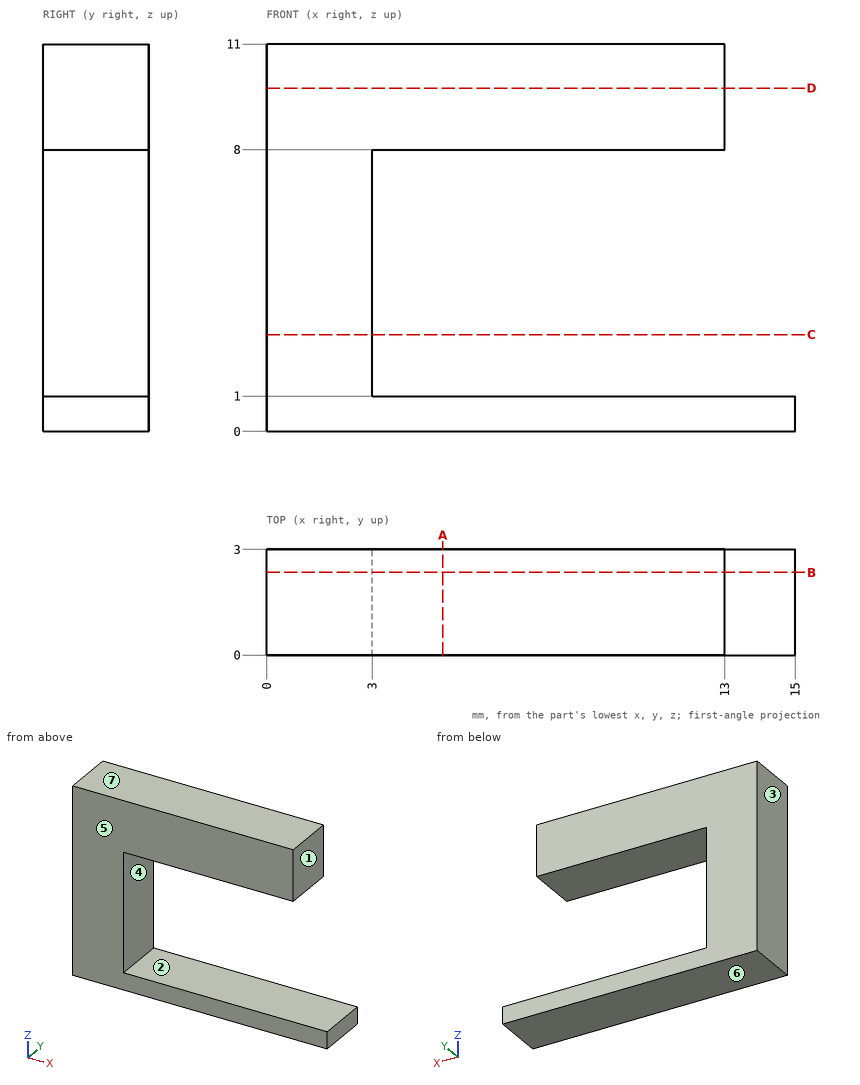
Geometry check sheet. Reference: drawing and pictorial views, mm from the part's lowest x, y, z. A direction names the side the tool comes from. Round coordinates to 2 decimals unless told otherwise and drop trailing zeros. Loops run counter-clockwise (first coordinate to the right, second up) from the corner with the lowest first, then second, coordinate; pieces in that order, holes last. Notation, with made-up numbers: (-27.5, 38.5) - (-3.5, 38.5) arc R25 ccw to (-3.5, 61.5) - close; hole circle Ø3 at (64.5, 88). An arc over 180 degrees is marked (long way). Use a Markdown table: item, result.
Q1. Cross-section at B-B on y = 2.35. Record the cut outline in (x, z).
Solutions:
| item | result |
|---|---|
| outline | (0, 0) - (15, 0) - (15, 1) - (3, 1) - (3, 8) - (13, 8) - (13, 11) - (0, 11) - close |
Q2. Go/stop test with a flat-tipped pin: P1, Ø0.9, axis at y = 2, z = 9.5, coming from the +X side. Record where the tip stops, or that it passes through.
Solutions:
| item | result |
|---|---|
| P1 | stops at x = 13 |
Q3. Cross-section at D-D on z = 9.75. Record the cut outline in (x, y).
Solutions:
| item | result |
|---|---|
| outline | (0, 0) - (13, 0) - (13, 3) - (0, 3) - close |
Q4. Cross-section at C-C on z = 2.75. Record the cut outline in (x, y), plus the area to 3 significant figures.
Solutions:
| item | result |
|---|---|
| outline | (0, 0) - (3, 0) - (3, 3) - (0, 3) - close |
| area | 9.00 mm2 |
Q5. Draft check along Z on the marked faces 4, 5, 6 and 7. Enter one of: released by +Z, released by -Z, zero draft, split by the parting line, or undercut.
Solutions:
| item | result |
|---|---|
| face 4 | undercut |
| face 5 | zero draft |
| face 6 | released by -Z |
| face 7 | released by +Z |
Q6. Access from +Z, -Z, +X, -X, +Y, -Y to the whole of each face (thin tool, end or side, straight path). Record for the marked faces 1, 2 and 3.
Solutions:
| item | result |
|---|---|
| face 1 | +Z, +X, +Y, -Y |
| face 2 | +X, +Y, -Y |
| face 3 | +Z, -Z, -X, +Y, -Y |
Q7. Cross-section at A-A on x = 5. Record the cut outline in (y, z).
Solutions:
| item | result |
|---|---|
| outline | (0, 0) - (3, 0) - (3, 1) - (0, 1) - close; (0, 8) - (3, 8) - (3, 11) - (0, 11) - close |
Q8. Material ranges on line 1 (Z direction, x = 7, y = 0.55); line 2 (X direction, y = 2.2, z = 8.5); line 3 (X direction, y = 2.65, z = 2.75), recorded low to high.
Solutions:
| item | result |
|---|---|
| line 1 | z = 0 to 1, 8 to 11 |
| line 2 | x = 0 to 13 |
| line 3 | x = 0 to 3 |
